```python
from build123d import *

# Parameters (mm, degrees)
SKETCH2_R             = 30
ACRYLICBASE_DEPTH     = 2
F_8_CLEARANCE_HOLE2_D = 4.3053


with BuildPart() as part:
    # Sketch2 → AcrylicBase (new body)
    with BuildSketch(Plane(origin=(0, 0, 0), x_dir=(1, 0, 0), z_dir=(0, 1, 0))):
        with Locations(Location((0, 0, 0), (0, 0, 270))):
            Circle(SKETCH2_R)
    extrude(amount=-ACRYLICBASE_DEPTH)

    # 8 Clearance Hole2 (through all)
    with Locations(Plane(origin=(0, 0, 0), x_dir=(-1, 0, 0), z_dir=(0, 1, 0))):
        with Locations((17.5, -17.5), (-17.5, -17.5), (-17.5, 17.5), (17.5, 17.5)):
            Hole(F_8_CLEARANCE_HOLE2_D / 2)


solid = part.part
```
Here's how the part is built. I have some questions about the finished solid (model axes, mm). Coordinates: 2 decimals unless noted, no trailing zeros. Order: outer loops, then holes, each group sorted by start corner. A loop starts at its lowest first (then second) coordinate and runs counter-clockwise, first axis right, second up. Notation, with made-up numbers: (69, 48) -> (123, 48) arc R23 ccw to (123, 84) -> close; hole circle Ø4 at (33, 36). An arc over 180 degrees is marked (long way). Return JSON: item names as keys, results as strings.
1) If we section it at A-A on y = -0.5: List the corners of the cut face in (x, z) for me.
Conclusion:
{"outline": "circle Ø60 at (0, 0); hole circle Ø4.31 at (-17.5, -17.5); hole circle Ø4.31 at (-17.5, 17.5); hole circle Ø4.31 at (17.5, -17.5); hole circle Ø4.31 at (17.5, 17.5)"}
2) I'm going to push flat-ended pins straight in: P1, Ø1, axis at y = -1.5, z = -4, coming from the -X side; P2, Ø3.5, axis at x = 17.5, z = -17.5, coming from the +Y side; P3, Ø5.5, axis at x = 17.5, z = 17.5, coming from the -Y side. Where does each tip first touch, or does it pass through?
Conclusion:
{"P1": "stops at x = -29.8", "P2": "passes through", "P3": "stops at y = -2"}
3) If I drill on probe 1 along X at (y, z) = (-1.3, 16.5); probe 2 along Z at (x, y) = (17.5, -0.95); probe 3 along Z at (x, y) = (-17, -1.85), over which ranges is the centre line in solid material (lowest first)?
Conclusion:
{"probe 1": "x = -25.05 to -19.41, -15.59 to 15.59, 19.41 to 25.05", "probe 2": "z = -24.37 to -19.65, -15.35 to 15.35, 19.65 to 24.37", "probe 3": "z = -24.72 to -19.59, -15.41 to 15.41, 19.59 to 24.72"}
4) If we section it at D-D on x = 24.5: List the corners of the cut face in (y, z) for me.
Conclusion:
{"outline": "(-2, -17.31) -> (0, -17.31) -> (0, 17.31) -> (-2, 17.31) -> close"}
5) If we section it at C-C on z = -17.5: List the corners of the cut face in (x, y) for me.
Conclusion:
{"outline": "(-24.37, -2) -> (-19.65, -2) -> (-19.65, 0) -> (-24.37, 0) -> close; (-15.35, -2) -> (15.35, -2) -> (15.35, 0) -> (-15.35, 0) -> close; (19.65, -2) -> (24.37, -2) -> (24.37, 0) -> (19.65, 0) -> close"}
6) Thinking about a two-plate mould opening in Z: for faces 1 (the cylindrical face through (17.22, -1.014, 19.634)), 2 (the cylindrical face through (-17.78, -1.014, 19.634)), 3 (the cylindrical face through (1.32, -0.99, -29.97)), 4 (the flat face through (0, 0, 0)), which applies, +Z half, -Z half, draft (parallel to the pull), parting line (faces both ways), or undercut?
Conclusion:
{"face 1": "undercut", "face 2": "undercut", "face 3": "parting line", "face 4": "draft"}
7) If we section it at B-B on x = -17.5: List the corners of the cut face in (y, z) for me, plus the area to 3 significant figures.
Conclusion:
{"outline": "(-2, -24.37) -> (0, -24.37) -> (0, -19.65) -> (-2, -19.65) -> close; (-2, -15.35) -> (0, -15.35) -> (0, 15.35) -> (-2, 15.35) -> close; (-2, 19.65) -> (0, 19.65) -> (0, 24.37) -> (-2, 24.37) -> close", "area": "80.2 mm²"}
